Geometry: final body of the model. Coordinates: model frame, mm. Round coordinates to 2 decimals unless told otherwise and drop trailing zeros. Order: outer loops, then holes, each group sorted by start corner. A loop starts at its lowest first (then second) coordinate and runs counter-clockwise, first axis right, second up. Notation, with made-up numbers: M 39.25,53 L 46.25,53 A24 cw 46.25,72 Z; hole C 80,36.5 d2. An arc over 180 degrees is marked long. Return JSON: item names as keys, results as strings. Group by question number.
Q1. Cut plane B-B on z = -111. Output: boundary loops of the cut face in (x, y).
Q2. Cut plane A-A on y = 12.7. Output: boundary loops of the cut face in (x, z) (3 decimals), and give its area (3 significant figures).
Q3. Contact query for flat-ended pins moving along their axis: pin 1 (5.5 mm diameter, centred on x = 9.13, y = 12.7, fed in from -Z); pin 2 (1.5 mm diameter, centred on x = 8.5, z = -81, fed in from +Y); pin 3 (6 mm diameter, centred on y = 6.5, z = -45, fed in from -X); pin 4 (1.1 mm diameter, centred on y = 14.5, z = 297.5, fed in from +X). Output: stop coordinate, or through.
Q4. Ray query, probe 1 along Z at (x, y) = (9.25, 8.5); probe 2 along Y at (x, z) = (15.5, 218); probe 3 along X at (y, z) = (17, 259). Return the intervals inside material, ascending.
Autodesk Inventor part; units mm, degrees
ref_plane "YZ Plane" through (0, 0, 0) normal (1, 0, 0) x (0, 1, 0)
ref_plane "XZ Plane" through (0, 0, 0) normal (0, 1, 0) x (-1, 0, 0)
ref_plane "XY Plane" through (0, 0, 0) normal (0, 0, 1) x (1, 0, 0)
sketch "Sketch1" plane through (0, 0, 0) normal (0, 0, 1) x (1, 0, 0)
  line L0 (0, 0) -> (19.05, 0)
  line L1 (19.05, 0) -> (19.05, 19.05)
  line L2 (19.05, 19.05) -> (18.2563, 19.05)
  line L3 (18.2563, 19.05) -> (18.2563, 0.7938)
  line L4 (18.2563, 0.7938) -> (0, 0.7937)
  line L5 (0, 0.7937) -> (0, 0)
  dimension "d0" = 19.05
  dimension "d1" = 19.05
  dimension "d2" = 0.7937
extrude "Extrusion1" add sketch "Sketch1" along normal blind 298.45
sketch "Sketch2" plane through (0, 0, 298.45) normal (0, 0, 1) x (1, 0, 0)
  line L0 (0, 0) -> (19.05, 0)
  line L1 (19.05, 0) -> (19.05, 19.05)
  line L2 (19.05, 19.05) -> (18.2563, 19.05)
  line L3 (18.2563, 19.05) -> (18.2563, 0.7938)
  line L4 (18.2563, 0.7938) -> (18.2563, 0)
extrude "Extrusion2" cut sketch "Sketch2" against normal blind 3.175
sketch "Sketch3" plane through (18.2563, 0, 297.6562) normal (0, 0, 1) x (1, 0, 0)
  line L0 (-18.2563, 0) -> (0, 0)
  line L1 (0, 0) -> (0, 19.05)
  line L2 (0, 19.05) -> (-18.2563, 19.05)
  line L3 (-18.2563, 19.05) -> (-18.2563, 0)
edge flange "Flange1" height 19.05 angle 90 thickness 0.7937 bend radius 0.635 thickness toward (0, 0, 1) relief straight relief width 0.7937 relief depth 0.3969 edges at (9.1281, 0.7938, 298.45) wall of the first edge with corners at (0, 0, 297.6562) (18.2563, 0, 297.6562) (18.2562, 19.05, 297.6562) (0, 19.05, 297.6562)
bend "Bend1"
corner "Corner1"
sketch "Sketch4" plane through (0, 19.05, 298.45) normal (0, 0, 1) x (1, 0, 0)
  line L0 (18.2563, 0) -> (18.2563, -17.6213)
  line L1 (0, -17.6213) -> (0, 0)
  line L2 (0, -6.35) -> (18.2563, -6.35) construction
  circle A0 centre (9.1281, -6.35) radius 3.3782
  point P0 (0, -19.05)
  dimension "d17" = 12.7
  dimension "d18" = 6.7564
extrude "Extrusion3" cut sketch "Sketch4" against normal through all
mirror "Mirror1" about plane through (13.8989, 5.1511, 0) normal (0, 0, -1)
equation "\"d7\" = BendReliefWidth"
equation "\"d8\" = BendReliefDepth"
equation "\"d9\" = MinimumRemnant"
equation "\"d10\" = BendRadius"
equation "\"d14\" = CornerReliefSize"
equation "\"d15\" = GapSize"
equation "\"d16\" = JacobiRadiusSize"
equation "\"BendRadius\" = Thickness"
equation "\"BendReliefWidth\" = Thickness"
equation "\"BendReliefDepth\" = 0.5 * Thickness"
equation "\"CornerReliefSize\" = 4 * Thickness"
equation "\"MinimumRemnant\" = 2 * Thickness"
equation "\"TransitionRadius\" = BendRadius"
equation "\"JacobiRadiusSize\" = Thickness"
equation "\"GapSize\" = Thickness"
properties part number "Chassis Back Electronics Protector Bar" material "Aluminum 6061"
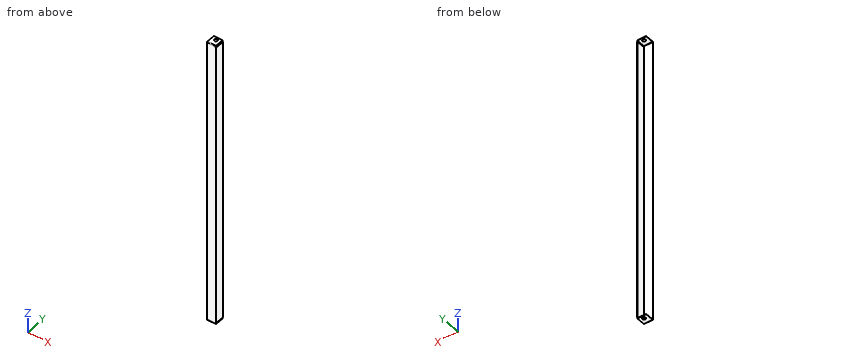
Result sheet:
{
 "1": {"outline": "M 0,0 L 19.05,0 L 19.05,19.05 L 18.26,19.05 L 18.26,0.79 L 0,0.79 Z"},
 "2": {"outline": "M 0,-298.45 L 5.75,-298.45 L 5.75,-297.656 L 0,-297.656 Z; M 0,297.656 L 5.75,297.656 L 5.75,298.45 L 0,298.45 Z; M 12.506,-298.45 L 18.256,-298.45 L 18.256,-297.656 L 12.506,-297.656 Z; M 12.506,297.656 L 18.256,297.656 L 18.256,298.45 L 12.506,298.45 Z; M 18.256,-295.275 L 19.05,-295.275 L 19.05,295.275 L 18.256,295.275 Z", "area": "487 mm²"},
 "3": {"pin 1": "passes through", "pin 2": "stops at y = 0.79", "pin 3": "stops at x = 18.26", "pin 4": "stops at x = 18.26"},
 "4": {"probe 1": "z = -298.45 to -297.66, 297.66 to 298.45", "probe 2": "y = 0 to 0.79", "probe 3": "x = 18.26 to 19.05"}
}
